from build123d import *

# Parameters (mm, degrees)
SKETCH1_W           = 143
SKETCH1_H           = 176
SKETCH1_W_2         = 78.5
SKETCH1_H_2         = 51.5
BOSS_EXTRUDE1_DEPTH = 2
SKETCH2_W           = 1
SKETCH2_H           = 1
CUT_EXTRUDE1_DEPTH  = 0.1
FILLET1_R           = 3


with BuildPart() as part:
    # Sketch1 → Boss-Extrude1 (new body)
    with BuildSketch(Plane(origin=(0, 0, 0), x_dir=(1, 0, 0), z_dir=(0, 1, 0))):
        with Locations((-31.5, -3)):
            Rectangle(SKETCH1_W, SKETCH1_H)
        with Locations((-46.5, 40)):
            Rectangle(SKETCH1_W_2, SKETCH1_H_2, mode=Mode.SUBTRACT)
        with BuildLine():
            Line((-64, -77), (-29, -77))
            ThreePointArc((-29, -77), (-28, -76), (-29, -75))
            Line((-29, -75), (-64, -75))
            ThreePointArc((-64, -75), (-65, -76), (-64, -77))
        make_face(mode=Mode.SUBTRACT)
        with BuildLine():
            Line((7.5, -70), (32.5, -70))
            ThreePointArc((32.5, -70), (33.5, -71), (32.5, -72))
            Line((32.5, -72), (7.5, -72))
            ThreePointArc((7.5, -72), (6.5, -71), (7.5, -70))
        make_face(mode=Mode.SUBTRACT)
        with BuildLine():
            Line((7.5, -76), (32.5, -76))
            ThreePointArc((32.5, -76), (33.5, -75), (32.5, -74))
            Line((32.5, -74), (7.5, -74))
            ThreePointArc((7.5, -74), (6.5, -75), (7.5, -76))
        make_face(mode=Mode.SUBTRACT)
        with BuildLine():
            Line((7.5, -66), (32.5, -66))
            ThreePointArc((32.5, -66), (33.5, -67), (32.5, -68))
            Line((32.5, -68), (7.5, -68))
            ThreePointArc((7.5, -68), (6.5, -67), (7.5, -66))
        make_face(mode=Mode.SUBTRACT)
        with BuildLine():
            Line((7.5, -62), (32.5, -62))
            ThreePointArc((32.5, -62), (33.5, -63), (32.5, -64))
            Line((32.5, -64), (7.5, -64))
            ThreePointArc((7.5, -64), (6.5, -63), (7.5, -62))
        make_face(mode=Mode.SUBTRACT)
        with BuildLine():
            Line((7.5, -58), (32.5, -58))
            ThreePointArc((32.5, -58), (33.5, -59), (32.5, -60))
            Line((32.5, -60), (7.5, -60))
            ThreePointArc((7.5, -60), (6.5, -59), (7.5, -58))
        make_face(mode=Mode.SUBTRACT)
        with BuildLine():
            Line((7.5, -40), (32.5, -40))
            ThreePointArc((32.5, -40), (33.5, -41), (32.5, -42))
            Line((32.5, -42), (7.5, -42))
            ThreePointArc((7.5, -42), (6.5, -41), (7.5, -40))
        make_face(mode=Mode.SUBTRACT)
        with BuildLine():
            Line((7.5, -46), (32.5, -46))
            ThreePointArc((32.5, -46), (33.5, -45), (32.5, -44))
            Line((32.5, -44), (7.5, -44))
            ThreePointArc((7.5, -44), (6.5, -45), (7.5, -46))
        make_face(mode=Mode.SUBTRACT)
        with BuildLine():
            Line((7.5, -36), (32.5, -36))
            ThreePointArc((32.5, -36), (33.5, -37), (32.5, -38))
            Line((32.5, -38), (7.5, -38))
            ThreePointArc((7.5, -38), (6.5, -37), (7.5, -36))
        make_face(mode=Mode.SUBTRACT)
        with BuildLine():
            Line((7.5, -32), (32.5, -32))
            ThreePointArc((32.5, -32), (33.5, -33), (32.5, -34))
            Line((32.5, -34), (7.5, -34))
            ThreePointArc((7.5, -34), (6.5, -33), (7.5, -32))
        make_face(mode=Mode.SUBTRACT)
        with BuildLine():
            Line((7.5, -28), (32.5, -28))
            ThreePointArc((32.5, -28), (33.5, -29), (32.5, -30))
            Line((32.5, -30), (7.5, -30))
            ThreePointArc((7.5, -30), (6.5, -29), (7.5, -28))
        make_face(mode=Mode.SUBTRACT)
        with BuildLine():
            Line((7.5, -10), (32.5, -10))
            ThreePointArc((32.5, -10), (33.5, -11), (32.5, -12))
            Line((32.5, -12), (7.5, -12))
            ThreePointArc((7.5, -12), (6.5, -11), (7.5, -10))
        make_face(mode=Mode.SUBTRACT)
        with BuildLine():
            Line((7.5, -16), (32.5, -16))
            ThreePointArc((32.5, -16), (33.5, -15), (32.5, -14))
            Line((32.5, -14), (7.5, -14))
            ThreePointArc((7.5, -14), (6.5, -15), (7.5, -16))
        make_face(mode=Mode.SUBTRACT)
        with BuildLine():
            Line((7.5, -6), (32.5, -6))
            ThreePointArc((32.5, -6), (33.5, -7), (32.5, -8))
            Line((32.5, -8), (7.5, -8))
            ThreePointArc((7.5, -8), (6.5, -7), (7.5, -6))
        make_face(mode=Mode.SUBTRACT)
        with BuildLine():
            Line((7.5, -2), (32.5, -2))
            ThreePointArc((32.5, -2), (33.5, -3), (32.5, -4))
            Line((32.5, -4), (7.5, -4))
            ThreePointArc((7.5, -4), (6.5, -3), (7.5, -2))
        make_face(mode=Mode.SUBTRACT)
        with BuildLine():
            Line((7.5, 2), (32.5, 2))
            ThreePointArc((32.5, 2), (33.5, 1), (32.5, 0))
            Line((32.5, 0), (7.5, 0))
            ThreePointArc((7.5, 0), (6.5, 1), (7.5, 2))
        make_face(mode=Mode.SUBTRACT)
        with BuildLine():
            Line((7.5, 20), (32.5, 20))
            ThreePointArc((32.5, 20), (33.5, 19), (32.5, 18))
            Line((32.5, 18), (7.5, 18))
            ThreePointArc((7.5, 18), (6.5, 19), (7.5, 20))
        make_face(mode=Mode.SUBTRACT)
        with BuildLine():
            Line((7.5, 14), (32.5, 14))
            ThreePointArc((32.5, 14), (33.5, 15), (32.5, 16))
            Line((32.5, 16), (7.5, 16))
            ThreePointArc((7.5, 16), (6.5, 15), (7.5, 14))
        make_face(mode=Mode.SUBTRACT)
        with BuildLine():
            Line((7.5, 24), (32.5, 24))
            ThreePointArc((32.5, 24), (33.5, 23), (32.5, 22))
            Line((32.5, 22), (7.5, 22))
            ThreePointArc((7.5, 22), (6.5, 23), (7.5, 24))
        make_face(mode=Mode.SUBTRACT)
        with BuildLine():
            Line((7.5, 28), (32.5, 28))
            ThreePointArc((32.5, 28), (33.5, 27), (32.5, 26))
            Line((32.5, 26), (7.5, 26))
            ThreePointArc((7.5, 26), (6.5, 27), (7.5, 28))
        make_face(mode=Mode.SUBTRACT)
        with BuildLine():
            Line((7.5, 32), (32.5, 32))
            ThreePointArc((32.5, 32), (33.5, 31), (32.5, 30))
            Line((32.5, 30), (7.5, 30))
            ThreePointArc((7.5, 30), (6.5, 31), (7.5, 32))
        make_face(mode=Mode.SUBTRACT)
    extrude(amount=BOSS_EXTRUDE1_DEPTH)

    # Sketch2 → Cut-Extrude1 (cut)
    with BuildSketch(Plane(origin=(0, 2, 0), x_dir=(1, 0, 0), z_dir=(0, 1, 0))):
        with Locations((-79.5, -34.5)):
            Rectangle(SKETCH2_W, SKETCH2_H)
    extrude(amount=-CUT_EXTRUDE1_DEPTH, mode=Mode.SUBTRACT)

    # Fillet1
    fillet1_edges = [part.edges().sort_by_distance(p)[0] for p in [
        (-103, 1, -85),
        (40, 1, -85),
        (40, 1, 91),
        (-103, 1, 91),
    ]]
    fillet(fillet1_edges, radius=FILLET1_R)


solid = part.part
CAD build for the part. Positions are in the model's coordinates, mm. Coordinates: 2 decimals unless noted, no trailing zeros. Order: outer loops, then holes, each group sorted by start corner. A loop starts at its lowest first (then second) coordinate and runs counter-clockwise, first axis right, second up.
Item 1: Band-saw the part on A-A on z = -37.5. List the corners of the cut face in (x, y), plus the area to 3 significant figures.
Check sheet entries:
outline: (-103, 0) - (-85.75, 0) - (-85.75, 2) - (-103, 2) - close; (-7.25, 0) - (40, 0) - (40, 2) - (-7.25, 2) - close
area: 129 mm2
Item 2: Band-saw the part on C-C on x = 16. Give the number of separate pieces and of enclosed holes in the cut face, plus the area to 3 significant figures.
Check sheet entries:
separate pieces: 21
enclosed holes: 0
area: 272 mm2
Item 3: Drill centre lines: L1, parallel to Z at x = -39.5, y = 0.6; L2, parallel to Z at x = -22.5, y = 0.7; L3, parallel to Z at x = -28.5, y = 1.4. Where is each one in solid material? Low to high.
Check sheet entries:
L1: z = -85 to -65.75, -14.25 to 75, 77 to 91
L2: z = -85 to -65.75, -14.25 to 91
L3: z = -85 to -65.75, -14.25 to 75.13, 76.87 to 91
Item 4: Band-saw the part on B-B on x = -53.5. List the corners of the cut face in (y, z), plus the area to 3 significant figures.
Check sheet entries:
outline: (0, -85) - (2, -85) - (2, -65.75) - (0, -65.75) - close; (0, -14.25) - (2, -14.25) - (2, 75) - (0, 75) - close; (0, 77) - (2, 77) - (2, 91) - (0, 91) - close
area: 245 mm2
